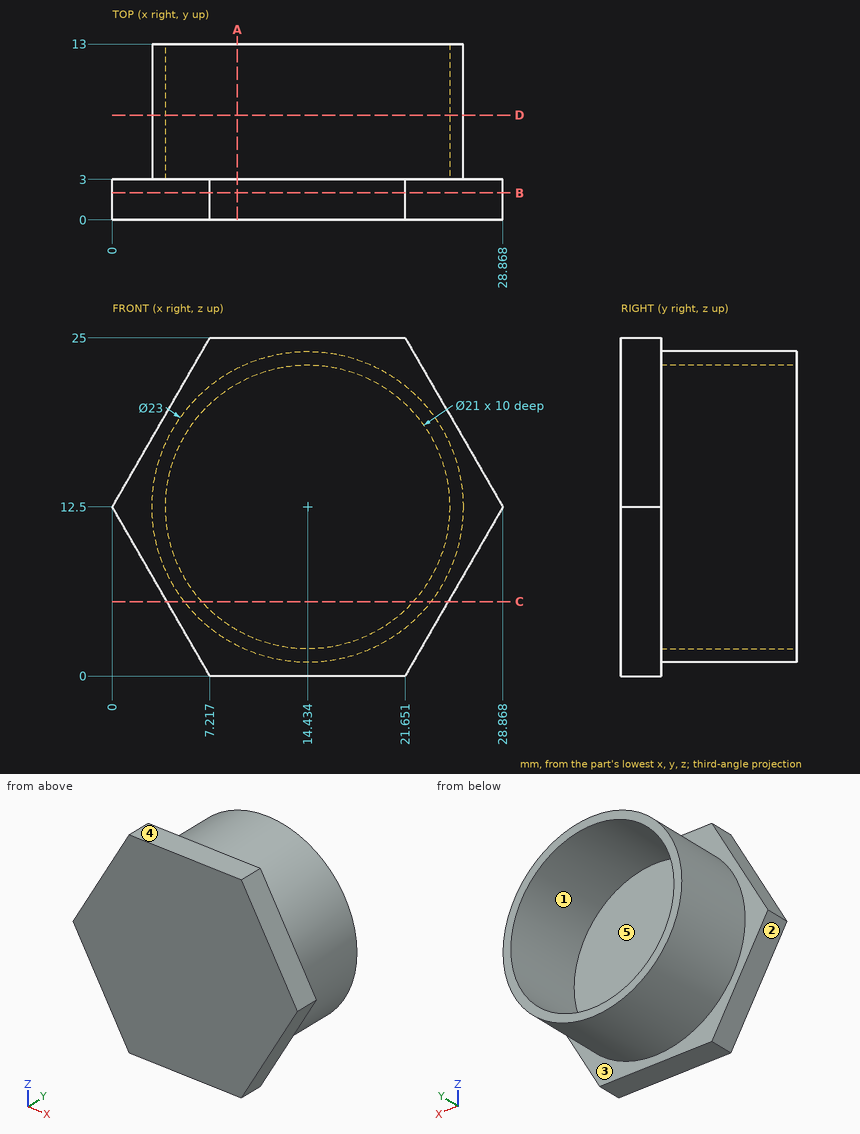
Verification items for this drawing (mm, ordinates from the low corner). A direction names the side the tool comes from. Coordinates: 2 decimals unless noted, no trailing zeros. Order: outer loops, then holes, each group sorted by start corner. A loop starts at its lowest first (then second) coordinate and runs counter-clockwise, first axis right, second up. Notation, with made-up numbers: (59.25, -6.5) -> (108.25, -6.5) arc R13 ccw to (108.25, 11.5) -> close; hole circle Ø1 at (75.5, -28.75). An arc over 180 degrees is marked (long way). Put each result on its own line as item: value. Start each with the question number.
1. Access from +Z, -Z, +X, -X, +Y, -Y to the whole of each face (thin tool, end or side, straight path). Record for the marked faces 4 and 5.
2. Cross-section at A-A, the plane x = 9.25. Record the boundary of the cut face in (y, z) (1 decimal).
3. Cross-section at C-C, the plane z = 5.5. Record the boundary of the cut face in (x, y).
4. Go/stop test with flat-tipped pins: pin 1 Ø2 at (y, z) = (8.5, 10) entering from +X (1 decimal); pin 2 Ø3 at (y, z) = (7, 10.5) entering from -X (1 decimal); pin 3 Ø6 at (y, z) = (6, 5) entering from -X. Record where each tip stops, or that it passes through.
5. Mould release check, pull along Z, two halves, no side actions. Record for the marked faces 1, 2 and 3: released by +Z, released by -Z, zero draft, split by the parting line, or undercut.
6. Cross-section at D-D, the plane y = 7.75. Record the boundary of the cut face in (x, z).
7. Material ranges on L1, parallel to X at y = 8, z = 15.5 (1 decimal); L2, parallel to Z at x = 12.75, y = 11 (1 decimal); L3, parallel to Z at x = 6, y = 8 (1 decimal), recorded low to high. Write a range as [from, to].
8. Cross-section at B-B, the plane y = 2. Record the boundary of the cut face in (x, z), then the cut area to 3 significant figures.
Computed:
1. face 4: +Z, +X, -X, +Y, -Y
1. face 5: +Y
2. outline: (0, 0) -> (3, 0) -> (3, 2.2) -> (13, 2.2) -> (13, 3.4) -> (3, 3.4) -> (3, 21.6) -> (13, 21.6) -> (13, 22.8) -> (3, 22.8) -> (3, 25) -> (0, 25) -> close
3. outline: (4.04, 0) -> (24.83, 0) -> (24.83, 3) -> (23.56, 3) -> (23.56, 13) -> (22.26, 13) -> (22.26, 3) -> (6.61, 3) -> (6.61, 13) -> (5.31, 13) -> (5.31, 3) -> (4.04, 3) -> close
4. pin 1: x = 25.8
4. pin 2: x = 2.9
4. pin 3: x = 3.85
5. face 1: undercut
5. face 2: released by -Z
5. face 3: zero draft
6. outline: circle Ø23 at (14.43, 12.5); hole circle Ø21 at (14.43, 12.5)
7. L1: [3.3, 4.4], [24.5, 25.5]
7. L2: [1.1, 2.1], [22.9, 23.9]
7. L3: [4.7, 6.2], [18.8, 20.3]
8. outline: (0, 12.5) -> (7.22, 0) -> (21.65, 0) -> (28.87, 12.5) -> (21.65, 25) -> (7.22, 25) -> close
8. area: 541 mm2
